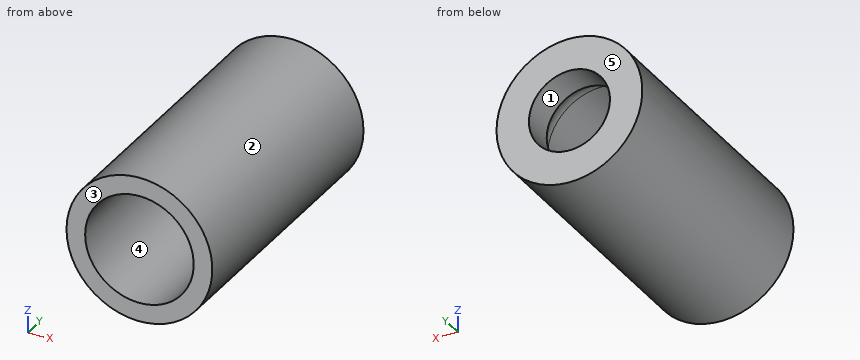
Autodesk Inventor part; units mm, degrees
ref_plane "YZ Plane" through (0, 0, 0) normal (1, 0, 0) x (0, 1, 0)
ref_plane "XZ Plane" through (0, 0, 0) normal (0, 1, 0) x (-1, 0, 0)
ref_plane "XY Plane" through (0, 0, 0) normal (0, 0, 1) x (1, 0, 0)
sketch "Sketch1" plane through (0, 0, 0) normal (0, 1, 0) x (-1, 0, 0)
  circle A0 centre (0, 0) radius 3.35
  circle A1 centre (0, 0) radius 4.5
  dimension "d0" = 6.7
  dimension "d1" = 9
extrude "Extrusion1" add sketch "Sketch1" along normal blind 15
sketch "Sketch2" plane through (0, 15, 0) normal (0, 1, 0) x (1, 0, 0)
  circle A0 centre (0, 0) radius 2.5
  circle A1 centre (0, 0) radius 3.35
  circle A2 centre (0, 0) radius 4.5
  dimension "d4" = 5
extrude "Extrusion2" add sketch "Sketch2" along normal blind 2 contours A1 | A2
fillet "Fillet1" radius 2 1 edges at (3.35, 15, 0)
equation "\"BendRadius\" = Thickness"
equation "\"BendReliefWidth\" = Thickness"
equation "\"BendReliefDepth\" = 0.5 * Thickness"
equation "\"CornerReliefSize\" = 4 * Thickness"
equation "\"MinimumRemnant\" = 2 * Thickness"
equation "\"TransitionRadius\" = BendRadius"
equation "\"JacobiRadiusSize\" = BendRadius"
equation "\"GapSize\" = Thickness"
properties part number "laser_tube_extender_single"
CAD build for the part. Positions are in the model's coordinates, mm. Face numbers are marked on the shaded views. A direction names the side the tool comes from. Round coordinates to 2 decimals unless told otherwise and drop trailing zeros. Loops run counter-clockwise (first coordinate to the right, second up) from the corner with the lowest first, then second, coordinate; pieces in that order, holes last. Notation, with made-up numbers: M 21,-19.75 L 46,-19.75 A21 cw 46,-15.75 Z; hole C -10,43 d1. An arc over 180 degrees is marked long. Use a Markdown table: item, result. Add a question column.
(1) Cut at A-A (y = 6.5). Give the cut face in (x, z).
(2) Which spindle directions (+Z, -Z, +X, -X, +Y, -Y) get a long thin tool onto all of the face, cutting with end or side? Do the marked faces 4 and 5. Say none if no direction does.
(3) Drill centre lines: line 1 (Z direction, x = 0, y = 3); line 2 (X direction, y = 16.4, z = 0). Where is each one in solid material? Low to high.
(4) Pull direction X, two halves, no side cores. Call the marked faces 1, 2 and 3: +X half, -X half, draft (parallel to the pull), parting line (faces both ways), or undercut.
(5) Flat gauge pins, fed straight in: pin 1 (1.5 mm diameter, centred on x = 3.5, y = 6, fed in from +Z); pin 2 (4 mm diameter, centred on y = 5, z = -3, fed in from +X); pin 3 (1 mm diameter, centred on x = 3, y = 5, fed in from +Z). Where does each tip first touch, or does it go through?
Geometry says:
| question | item | result |
|---|---|---|
| 1 | outline | C 0,0 d9; hole C 0,0 d6.7 |
| 2 | face 4 | -Y |
| 2 | face 5 | +Z, -Z, +X, -X, +Y |
| 3 | line 1 | z = -4.5 to -3.35, 3.35 to 4.5 |
| 3 | line 2 | x = -4.5 to -2.5, 2.5 to 4.5 |
| 4 | face 1 | undercut |
| 4 | face 2 | parting line |
| 4 | face 3 | draft |
| 5 | pin 1 | stops at z = 3.56 |
| 5 | pin 2 | stops at x = 4.39 |
| 5 | pin 3 | stops at z = 3.74 |
